Model file for the job. Use its own axes, mm. Face numbers are marked on the shaded views. A direction names the side the tool comes from. Give positions to 0.01 mm unless a question says otherwise; leave off trailing zeros. Order: outer loops, then holes, each group sorted by start corner. A loop starts at its lowest first (then second) coordinate and runs counter-clockwise, first axis right, second up. Notation, with made-up numbers: M -24,3.5 L 3,3.5 A24 cw 3,30.5 Z; hole C 13.25,-15.5 d3. An arc over 180 degrees is marked long. Return JSON: item names as keys, results as strings. Group by question number.
1. 3-axis set-ups, long thin cutter, end or side, ignore diameter. For the marked faces 1, 2 and 3: which of +Z, -Z, +X, -X, +Y, -Y reach the whole face in a straight line?
2. Slice it at D-D on x = 3.5. List the corners of the cut face in (y, z).
3. Slice it at C-C on z = -1.15. List the corners of the cut face in (x, y).
4. Slice it at B-B on x = -1.5. List the corners of the cut face in (y, z), then the cut area to 3 significant figures.
5. Pin check, flat tips, straight feed: pin 1 (2 mm diameter, centred on x = 4, z = -2, fed in from +Y); pin 2 (5 mm diameter, centred on x = 1, y = 5.5, fed in from -Z); pin 3 (3 mm diameter, centred on x = 2.5, z = -0.5, fed in from -Y); pin 4 (2 mm diameter, centred on y = 2, z = 2, fed in from +X). Stop position of each tip, or through.
6. Wall check: probe 1 along X at (y, z) = (-2.5, -1.05); probe 2 along X at (y, z) = (-3, -0.75); probe 3 along X at (y, z) = (-2, 2.15). Give the ranges that are in metal, low to high. Write a range as [from, to].
7. Slice it at A-A on y = -1.75. List the corners of the cut face in (x, z), then the cut area to 3 significant figures.
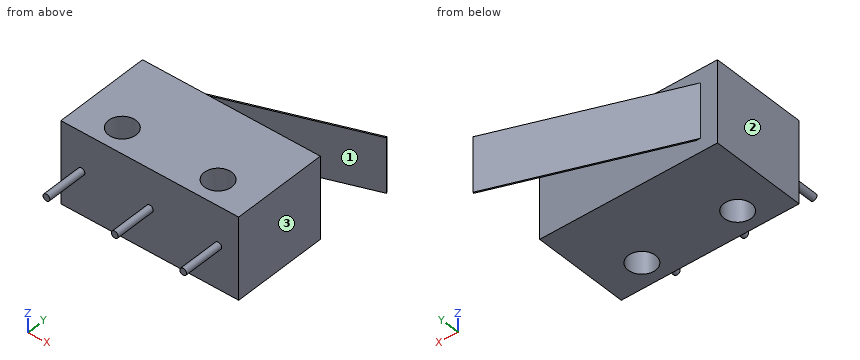
Autodesk Inventor part; units mm, degrees
ref_plane "YZ Plane" through (0, 0, 0) normal (1, 0, 0) x (0, 1, 0)
ref_plane "XZ Plane" through (0, 0, 0) normal (0, 1, 0) x (-1, 0, 0)
ref_plane "XY Plane" through (0, 0, 0) normal (0, 0, 1) x (1, 0, 0)
sketch "Boceto1" plane through (0, 0, 0) normal (0, 0, 1) x (1, 0, 0)
  line L0 (-6.5, 3.5) -> (6.5, 3.5)
  line L1 (6.5, 3.5) -> (6.5, -3.5)
  line L2 (6.5, -3.5) -> (-6.5, -3.5)
  line L3 (-6.5, -3.5) -> (-6.5, 3.5)
  line L4 (0, -4.9) -> (0, 4.9)
  line L5 (-9.1, 0) -> (9.1, 0)
  point P0 (0, 0)
  dimension "d0" = 13
  dimension "d1" = 7
extrude "Extrusión1" add sketch "Boceto1" along normal mid plane 6
sketch "Boceto2" plane through (0, 0, 3) normal (0, 0, 1) x (1, 0, 0)
  circle A0 centre (3.5, -1.75) radius 1
  circle A1 centre (-3.5, -1.75) radius 1
  line L0 (-6.5, 3.5) -> (-6.5, -3.5)
  line L1 (6.5, -3.5) -> (6.5, 3.5)
  line L2 (-6.5, -3.5) -> (6.5, -3.5)
  point P0 (0, 0)
  dimension "d4" = 2
  dimension "d5" = 2
  dimension "d6" = 3
  dimension "d8" = 3
  dimension "d25" = 1.75
  dimension "d26" = 1.75
extrude "Extrusión2" cut sketch "Boceto2" against normal up to surface (6 mm away)
sketch "Boceto3" plane through (0, 0, 0) normal (0, 0, 1) x (1, 0, 0)
  line L0 (-6.5, 3.5) -> (6.5, 3.5)
  line L1 (-6.5, 3.5) -> (-5.25, 3.5)
  line L2 (-5.25, 3.5) -> (7.4359, 8.1173)
  line L3 (7.4359, 8.1173) -> (7.4701, 8.0233)
  line L4 (7.4701, 8.0233) -> (-4.9576, 3.5)
  line L5 (-4.9576, 3.5) -> (-5.25, 3.5)
  point P0 (0, 0)
  dimension "d11" = 1.25
  dimension "d12" = 13.5
  dimension "d13" = 160
  dimension "d14" = 0.1
  dimension "d15" = 90
extrude "Extrusión3" add sketch "Boceto3" against normal mid plane 4
sketch "Boceto4" plane through (-6.5, -3.5, -3) normal (0, -1, 0) x (1, 0, 0)
  circle A0 centre (1.5, 3.1423) radius 0.25
  circle A1 centre (11.5, 3.1423) radius 0.25
  line L0 (0, 0) -> (0, 6)
  circle A2 centre (6.5, 3.1423) radius 0.25
  line L1 (13, 6) -> (13, 0)
  point P0 (6.5, 3)
  dimension "d18" = 1.5
  dimension "d20" = 0.5
  dimension "d21" = 0.5
  dimension "d22" = 0.5
  dimension "d27" = 1.5
extrude "Extrusión4" add sketch "Boceto4" along normal blind 3
equation "\"d5\" = d4"
equation "\"d26\" = d25"
equation "\"d21\" = d20"
equation "\"d22\" = d21"
properties part number "Micro Switch"
Result:
{
 "1": {"face 1": "+Z, -Z, +X", "face 2": "+Z, -Z, -X, +Y, -Y", "face 3": "+Z, -Z, +X, -Y"},
 "2": {"outline": "M -3.5,-3 L -2.75,-3 L -2.75,3 L -3.5,3 Z; M -0.75,-3 L 3.5,-3 L 3.5,3 L -0.75,3 Z; M 6.58,-2 L 6.68,-2 L 6.68,2 L 6.58,2 Z"},
 "3": {"outline": "M -6.5,-3.5 L 6.5,-3.5 L 6.5,3.5 L -4.96,3.5 L 7.47,8.02 L 7.44,8.12 L -5.25,3.5 L -6.5,3.5 Z; hole C -3.5,-1.75 d2; hole C 3.5,-1.75 d2"},
 "4": {"outline": "M -3.5,-3 L 3.5,-3 L 3.5,3 L -3.5,3 Z; M 4.76,-2 L 4.86,-2 L 4.86,2 L 4.76,2 Z", "area": "42.4 mm2"},
 "5": {"pin 1": "stops at y = 7.23", "pin 2": "stops at z = -3", "pin 3": "stops at y = -3.5", "pin 4": "stops at x = 6.5"},
 "6": {"probe 1": "x = [-6.5, -4.16], [-2.84, 2.84], [4.16, 6.5]", "probe 2": "x = [-6.5, 6.5]", "probe 3": "x = [-6.5, -4.47], [-2.53, 2.53], [4.47, 6.5]"},
 "7": {"outline": "M -6.5,-3 L -4.5,-3 L -4.5,3 L -6.5,3 Z; M -2.5,-3 L 2.5,-3 L 2.5,3 L -2.5,3 Z; M 4.5,-3 L 6.5,-3 L 6.5,3 L 4.5,3 Z", "area": "54.0 mm2"}
}
